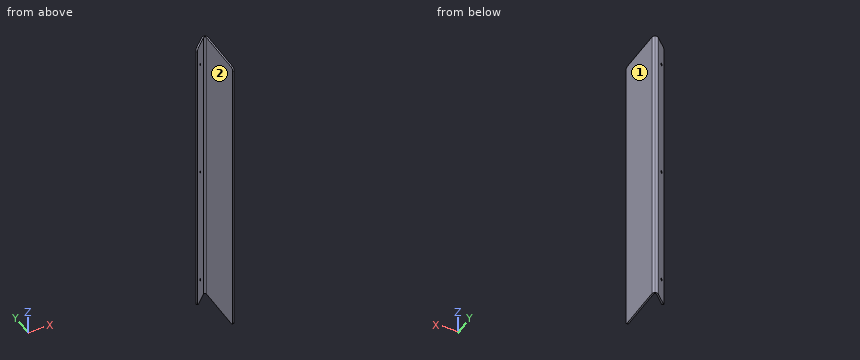
```python
from build123d import *

# Parameters (mm, degrees)
SKETCH1_W            = 590.55
SKETCH1_H            = 114.3
BASE_FLANGE1_DEPTH   = 3.175
EDGE_FLANGE1_START   = -590.55
EDGE_FLANGE1_DEPTH   = 590.55
EDGE_FLANGE1_2_DEPTH = 590.55
FILLET1_R            = 6.35
SKETCH9_R            = 2.45745
CUT_EXTRUDE1_DEPTH   = 3.18516


# Read off the part's stored shape, not the designer's step: Edge-Flange1
# Sheet-metal steps are written as plain solids
with BuildPart() as part:
    # Sketch1 → Base-Flange1 (new body)
    with BuildSketch(Plane(origin=(0, 0, 0), x_dir=(0, 0, -1), z_dir=(1, 0, 0))):
        with Locations((295.275, 57.15)):
            Rectangle(SKETCH1_W, SKETCH1_H)
    extrude(amount=-BASE_FLANGE1_DEPTH)

    # Edge-Flange1 outline → Edge-Flange1 (cut)
    with BuildSketch(Plane.XY.offset(EDGE_FLANGE1_START)):
        with BuildLine():
            Line((-3.175, 114.3), (-3.175, 107.644005193))
            ThreePointArc((-3.175, 107.644005193), (-0.850738686, 105.319743879), (0, 102.144743879))
            Line((0, 102.144743879), (0, 114.3))
            Line((0, 114.3), (-3.175, 114.3))
        make_face()
    extrude(amount=EDGE_FLANGE1_DEPTH, mode=Mode.SUBTRACT)

    # Edge-Flange1 2 outline → Edge-Flange1 2 (add)
    with BuildSketch(Plane.XY.offset(EDGE_FLANGE1_START)):
        with BuildLine():
            ThreePointArc((-3.175, 107.644005193), (-7.178841321, 108.440418748), (-10.840128061, 106.634871939))
            Line((-10.840128061, 106.634871939), (-35.921024484, 81.553975516))
            Line((-35.921024484, 81.553975516), (-33.675960454, 79.308911485))
            Line((-33.675960454, 79.308911485), (-8.59506403, 104.389807909))
            ThreePointArc((-8.59506403, 104.389807909), (-5.134980102, 105.078061395), (-3.175, 102.144743879))
            Line((-3.175, 102.144743879), (-3.175, 107.644005193))
        make_face()
    extrude(amount=EDGE_FLANGE1_2_DEPTH)

    # Fillet1
    fillet1_edges = [part.edges().sort_by_distance(p)[0] for p in [
        (-34.798492469, 80.4314435, 0),
        (-34.798492469, 80.4314435, -590.55),
        (-1.5875, 0, -590.55),
        (-1.5875, 0, 0),
    ]]
    fillet(fillet1_edges, radius=FILLET1_R)

    # Sketch9 → Cut-Extrude1 (cut)
    with BuildSketch(Plane(origin=(-58.7375, 58.7375, 0), x_dir=(0, 0, 1), z_dir=(-0.7071067811865465, 0.7071067811865487, 0))):
        with Locations(Location((-542.925, 48.687112999, 0), (0, 0, 270))):
            Circle(SKETCH9_R)
        with Locations(Location((-295.275, 48.687112999, 0), (0, 0, 270))):
            Circle(SKETCH9_R)
        with Locations(Location((-47.625, 48.687112999, 0), (0, 0, 270))):
            Circle(SKETCH9_R)
    extrude(amount=-CUT_EXTRUDE1_DEPTH, mode=Mode.SUBTRACT)


solid = part.part
```
Build history of the part. All positions in model axes, mm. Face numbers are marked on the shaded views. Round coordinates to 2 decimals unless told otherwise and drop trailing zeros. Write each loop counter-clockwise with the first axis right and the second up, starting at its lowest first coordinate (ties: lowest second). Pieces come first, ordered by that corner, then holes. Notation, with made-up numbers: (24.5, -5.5) - (83.5, -5.5) arc R12 ccw to (83.5, 4.5) - close; hole circle Ø2 at (37.25, 89.5). An arc over 180 degrees is marked (long way). Write each question's results on one line, items separated by ' | '. Start each with the question number.
Item 1: Drop flat-ended pins along their axis: P1, Ø10, axis at x = -6, y = 93, coming from the +Z side; P2, Ø6, axis at x = -16.5, z = -91.5, coming from the -Y side; P3, Ø3, axis at x = -4.5, z = -498.5, coming from the +Y side; P4, Ø12, axis at x = -27.5, z = -257, coming from the -Y side. Give the stop position or say it passes through.
Item 2: Mould opens along X. For the marked faces 1 and 2 say: pulls with the +X half, pulls with the -X half, needs draft (parallel to the pull), parting line crosses it, or undercut.
Item 3: Saw through at A-A (z = -69). Write the cut outline in (x, y) (3 decimals).
Item 4: Saw through at B-B (y = 41). Write the cut outline in (x, z) (3 decimals), and give its area (4 significant figures).
Item 5: Wall check: L1, parallel to Y at x = -5.5, z = -287.5; L2, parallel to X at y = 83, z = -456 (3 decimals); L3, parallel to X at y = 51, z = -47 (3 decimals). Give the ranges that are in metal, low to high. Write a range as [from, to].
Results are:
1) P1: stops at z = 0 | P2: stops at y = 93.48 | P3: stops at y = 108.49 | P4: stops at y = 79.48
2) face 1: pulls with the +X half | face 2: undercut
3) outline: (-35.921, 81.554) - (-33.676, 79.309) - (-8.595, 104.39) arc R3.175 cw to (-3.175, 102.145) - (-3.175, 0) - (0, 0) - (0, 102.145) arc R6.35 ccw to (-10.84, 106.635) - close
4) outline: (-3.175, -590.55) - (0, -590.55) - (0, 0) - (-3.175, 0) - close | area: 1,875 mm²
5) L1: y = [105.2, 108.44] | L2: x = [-34.475, -29.985], [-3.175, 0] | L3: x = [-3.175, 0]
